from build123d import *

# Parameters (mm, degrees)
F0_W     = 609.6
F0_H     = 152.4
F1_DEPTH = 355.6
F2_W     = 603.25
F2_H     = 146.05
F3_DEPTH = 352.425
F4_W     = 596.9
F4_H     = 139.7
F5_DEPTH = 352.425
F7_DEPTH = 25.4


with BuildPart() as f1:
    # F0 (on Front) → F1 (new body)
    with BuildSketch(Plane.XZ):
        Rectangle(F0_W, F0_H)
    extrude(amount=F1_DEPTH)

    # F2 (on face) → F3 (cut)
    with BuildSketch(Plane.XZ.offset(355.6)):
        Rectangle(F2_W, F2_H)
    extrude(amount=-F3_DEPTH, mode=Mode.SUBTRACT)

    # F4 (on face) → F5 (join, through all)
    with BuildSketch(Plane.XZ.offset(3.175)):
        Rectangle(F4_W, F4_H)
    extrude(amount=F5_DEPTH)

    # F6 (on face) → F7 (cut)
    with BuildSketch(Plane.XZ.offset(355.6)):
        with BuildLine():
            ThreePointArc((-101.6, 57.15), (-152.4, 6.35), (-101.6, -44.45))
            Line((-101.6, -44.45), (0, -44.45))
            Line((0, -44.45), (0, 57.15))
            Line((0, 57.15), (-101.6, 57.15))
        make_face()
        with BuildLine():
            Line((0, 57.15), (0, -44.45))
            Line((0, -44.45), (101.6, -44.45))
            ThreePointArc((101.6, -44.45), (152.4, 6.35), (101.6, 57.15))
            Line((101.6, 57.15), (0, 57.15))
        make_face()
    extrude(amount=-F7_DEPTH, mode=Mode.SUBTRACT)


solid = f1.part
Work out the finished part from the listing and answer in its coordinate system (mm). A direction names the side the tool comes from. Give positions to 0.01 mm unless a question says otherwise; leave off trailing zeros. Write each loop counter-clockwise with the first axis right and the second up, starting at its lowest first coordinate (ties: lowest second). Pieces come first, ordered by that corner, then holes. Notation, with made-up numbers: (77.25, 73) - (92.25, 73) arc R24 ccw to (92.25, 104) - close; hole circle Ø1 at (44, 57.5). An arc over 180 degrees is marked (long way). One line per item, written item: value. Start each with the question number.
1. Find section D-D (x = -46). Write down the section's boundary in (y, z) (3 decimals), then the cut area to 3 significant figures.
2. Find section A-A (y = -106). Write down the section's boundary in (x, z) (3 decimals).
3. Find section B-B (x = 218). Write down the section's boundary in (y, z) (3 decimals), then the cut area to 3 significant figures.
4. Find section C-C (z = 6.35). Write down the section's boundary in (x, y) (3 decimals), then the cut area to 3 significant figures.
5. Consider probe 1 along X at (y, z) = (-246.5, 67.5) (3 decimals); probe 2 along Z at (x, y) = (180.5, -15) (3 decimals); probe 3 along Y at (x, z) = (106, 24). Determine where each line is inside the solid, lowest interval first.
6. For faces 1 (the flat face through (-4, 0, 1)), 2 (the cylindrical face through (152.388, -343.078, 5.233)), determine the directions among +Z, -Z, +X, -X, +Y, -Y from which every point of the face is accessible in a straight line to the end or side of a thin tool.
7. For a pull along Z with two mould halves and no side action, classify faces 3 (the flat face through (-304.8, -175, -1)), 4 (the flat face through (-4, -177, -69.85)), 5 (the flat face through (-4, -182, -73.025)), 6 (the flat face through (-4, -175, 76.2)) as +Z half, -Z half, draft (parallel to the pull), parting line (faces both ways), or undercut.
Geometry results:
1. outline: (-355.6, -76.2) - (0, -76.2) - (0, 76.2) - (-355.6, 76.2) - (-355.6, 73.025) - (-3.175, 73.025) - (-3.175, 69.85) - (-355.6, 69.85) - (-355.6, 57.15) - (-330.2, 57.15) - (-330.2, -44.45) - (-355.6, -44.45) - (-355.6, -69.85) - (-3.175, -69.85) - (-3.175, -73.025) - (-355.6, -73.025) - close
1. area: 49,400 mm2
2. outline: (-304.8, -76.2) - (304.8, -76.2) - (304.8, 76.2) - (-304.8, 76.2) - close; (-298.45, -69.85) - (298.45, -69.85) - (298.45, 69.85) - (-298.45, 69.85) - close; hole (-301.625, -73.025) - (301.625, -73.025) - (301.625, 73.025) - (-301.625, 73.025) - close
3. outline: (-355.6, -76.2) - (0, -76.2) - (0, 76.2) - (-355.6, 76.2) - (-355.6, 73.025) - (-3.175, 73.025) - (-3.175, 69.85) - (-355.6, 69.85) - (-355.6, -69.85) - (-3.175, -69.85) - (-3.175, -73.025) - (-355.6, -73.025) - close
3. area: 52,000 mm2
4. outline: (-304.8, -355.6) - (-301.625, -355.6) - (-301.625, -3.175) - (-298.45, -3.175) - (-298.45, -355.6) - (-152.4, -355.6) - (-152.4, -330.2) - (152.4, -330.2) - (152.4, -355.6) - (298.45, -355.6) - (298.45, -3.175) - (301.625, -3.175) - (301.625, -355.6) - (304.8, -355.6) - (304.8, 0) - (-304.8, 0) - close
4. area: 207,000 mm2
5. probe 1: -304.8 to -301.625, -298.45 to 298.45, 301.625 to 304.8
5. probe 2: -76.2 to -73.025, -69.85 to 69.85, 73.025 to 76.2
5. probe 3: -330.2 to 0
6. face 1: +Z, -Z, +X, -X, +Y
6. face 2: -Y
7. face 3: draft
7. face 4: undercut
7. face 5: undercut
7. face 6: +Z half
